from build123d import *

# Parameters (mm, degrees)
SKETCH1_R           = 5.7
BOSS_EXTRUDE1_DEPTH = 8
SKETCH2_R           = 8.005
CUT_EXTRUDE1_DEPTH  = 2.1


with BuildPart() as part:
    # Sketch1 → Boss-Extrude1 (new body)
    with BuildSketch(Plane.XY):
        with BuildLine():
            Line((0, 14), (0, 22))
            Line((0, 22), (40.6, 22))
            Line((40.6, 22), (40.6, 14))
            Line((40.6, 14), (34.3, 14))
            ThreePointArc((34.3, 14), (31.3, 11), (34.3, 8))
            Line((34.3, 8), (40.6, 8))
            Line((40.6, 8), (40.6, 0))
            Line((40.6, 0), (0, 0))
            Line((0, 0), (0, 8))
            Line((0, 8), (6.3, 8))
            ThreePointArc((6.3, 8), (9.3, 11), (6.3, 14))
            Line((6.3, 14), (0, 14))
        make_face()
        with Locations((20.3, 11)):
            Circle(SKETCH1_R, mode=Mode.SUBTRACT)
    extrude(amount=BOSS_EXTRUDE1_DEPTH)

    # Sketch2 → Cut-Extrude1 (cut)
    with BuildSketch(Plane.XY.offset(8)):
        with Locations((20.3, 11)):
            Circle(SKETCH2_R)
    extrude(amount=-CUT_EXTRUDE1_DEPTH, mode=Mode.SUBTRACT)

    # Sketch3 → M3x0.5 Tapped Hole1 (revolve, cut)
    with BuildSketch(Plane(origin=(32.6, 22, 4), x_dir=(0, 0, 1), z_dir=(1, 0, 0))):
        Polygon((0, 0), (0, 5.751075774), (1.25, 5), (1.25, 0.275), (1.525, 0), align=None)
    m3x0_5_tapped_hole1 = revolve(axis=Axis((32.6, 28.35, 4), (0, -1, 0)), mode=Mode.SUBTRACT)

    # Mirror1: M3x0.5 Tapped Hole1 across plane
    add(m3x0_5_tapped_hole1.mirror(Plane(origin=(20.3, 0, 0), x_dir=(0, 0, 1), z_dir=(1, 0, 0))), mode=Mode.SUBTRACT)

    # Sketch5 → M3x0.5 Tapped Hole2 (revolve, cut)
    with BuildSketch(Plane(origin=(40.6, 18, 4), x_dir=(0, 0, -1), z_dir=(0, 1, 0))):
        Polygon((0, 0), (0, 7.251075774), (1.25, 6.5), (1.25, 0.275), (1.525, 0), align=None)
    m3x0_5_tapped_hole2 = revolve(axis=Axis((46.95, 18, 4), (-1, 0, 0)), mode=Mode.SUBTRACT)

    # Mirror2: M3x0.5 Tapped Hole2 across plane
    add(m3x0_5_tapped_hole2.mirror(Plane(origin=(0, 11, 0), x_dir=(0, 0, 1), z_dir=(0, -1, 0))), mode=Mode.SUBTRACT)

    # Mirror3: M3x0.5 Tapped Hole2 across plane
    add(m3x0_5_tapped_hole2.mirror(Plane(origin=(20.3, 0, 0), x_dir=(0, 0, 1), z_dir=(1, 0, 0))), mode=Mode.SUBTRACT)

    # Mirror3 copy 1 sketch → Mirror3 copy 1 (revolve, cut)
    with BuildSketch(Plane(origin=(0, 4, 4), x_dir=(0, 0, -1), z_dir=(0, -1, 0))):
        Polygon((0, 0), (0, 7.251075774), (1.25, 6.5), (1.25, 0.275), (1.525, 0), align=None)
    revolve(axis=Axis((-6.35, 4, 4), (1, 0, 0)), mode=Mode.SUBTRACT)


solid = part.part
Here's how the part is built. I have some questions about the finished solid (model axes, mm). A direction names the side the tool comes from. Give positions to 0.01 mm unless a question says otherwise; leave off trailing zeros. Loops run counter-clockwise (first coordinate to the right, second up) from the corner with the lowest first, then second, coordinate; pieces in that order, holes last. Notation, with made-up numbers: (46, 44.25) -> (66, 44.25) arc R19 cw to (66, 49.25) -> close; hole circle Ø9 at (51, 51.5). An arc over 180 degrees is marked (long way). Answer as a JSON object with one key per item and string values. Group by question number.
Item 1: Imagine slicing it at D-D on y = 12.75. Write out the boundary of the cut face in (x, z), then the cut area to 3 significant figures.
Item 2: Will these pins go through, and if not, where does the flat tip stop? pin 1 (2 mm diameter, centred on y = 18, z = 4, fed in from -X); pin 2 (13 mm diameter, centred on x = 20.3, y = 11, fed in from +Z); pin 3 (3 mm diameter, centred on y = 4, z = 4, fed in from -X) (3 decimals).
Item 3: On a 3-axis mill with a long thin cutter (end or side, diameter ignored), from which of +Z, -Z, +X, -X, +Y, -Y can I reach the whole of each face in a straight line? I mean faces 4 (the cylindrical face through (12.303, 11.352, 6.965)), 5 (the conical face through (33.48, 4.15, 4.16)), 6 (the flat face through (3, 14, 4)). Say none if no direction works.
Item 4: Thinking about a two-plate mould opening in Z: for faces 1 (the flat face through (26, 8, 5.9)), 2 (the conical face through (8.01, 16.38, 3.78)), 3 (the cylindrical face through (25.737, 12.712, 2.909)), which applies, pulls with the +Z half, pulls with the -Z half, needs draft (parallel to the pull), parting line crosses it, or undercut?
Item 5: Imagine slicing it at A-A on x = 37.5. Write out the boundary of the cut face in (y, z).
Item 6: Imagine slicing it at C-C on x = 20.3. Write out the boundary of the cut face in (y, z) (3 decimals).
Item 7: Imagine slicing it at B-B on z = 1.5. Write out the boundary of the cut face in (x, y), then the cut area to 3 significant figures.
Item 8: I need wall thicknesses on L1, parallel to Y at x = 38.5, z = 4; L2, parallel to Z at x = 38.25, y = 18; L3, parallel to Y at x = 20.3, z = 6.9 (3 decimals). Which ranges of each line are inside material? Lowest first, please.
Answer list:
{
 "1": {"outline": "(8.74, 0) -> (14.88, 0) -> (14.88, 5.9) -> (12.49, 5.9) -> (12.49, 8) -> (8.74, 8) -> close; (25.72, 0) -> (31.86, 0) -> (31.86, 8) -> (28.11, 8) -> (28.11, 5.9) -> (25.72, 5.9) -> close", "area": "88.2 mm2"},
 "2": {"pin 1": "stops at x = 6.65", "pin 2": "stops at z = 5.9", "pin 3": "stops at x = 0.025"},
 "3": {"face 4": "+Z", "face 5": "+X", "face 6": "+Z, -Z, -X"},
 "4": {"face 1": "pulls with the +Z half", "face 2": "undercut", "face 3": "needs draft"},
 "5": {"outline": "(0, 0) -> (8, 0) -> (8, 8) -> (0, 8) -> close; (14, 0) -> (22, 0) -> (22, 8) -> (14, 8) -> close; hole circle Ø2.5 at (4, 4); hole circle Ø2.5 at (18, 4)"},
 "6": {"outline": "(0, 0) -> (5.3, 0) -> (5.3, 5.9) -> (2.995, 5.9) -> (2.995, 8) -> (0, 8) -> close; (16.7, 0) -> (22, 0) -> (22, 8) -> (19.005, 8) -> (19.005, 5.9) -> (16.7, 5.9) -> close"},
 "7": {"outline": "(0, 0) -> (40.6, 0) -> (40.6, 8) -> (34.3, 8) arc R3 cw to (34.3, 14) -> (40.6, 14) -> (40.6, 22) -> (0, 22) -> (0, 14) -> (6.3, 14) arc R3 cw to (6.3, 8) -> (0, 8) -> close; hole circle Ø11.4 at (20.3, 11)", "area": "687 mm2"},
 "8": {"L1": "y = 0 to 2.75, 5.25 to 8, 14 to 16.75, 19.25 to 22", "L2": "z = 0 to 2.75, 5.25 to 8", "L3": "y = 0 to 2.995, 19.005 to 22"}
}
